Design review of the part built by this model. Coordinates are the model's own, in mm. Round coordinates to 2 decimals unless told otherwise and drop trailing zeros. Order: outer loops, then holes, each group sorted by start corner. A loop starts at its lowest first (then second) coordinate and runs counter-clockwise, first axis right, second up. Notation, with made-up numbers: M -16.75,36.5 L 16.25,36.5 A22 cw 16.25,74.5 Z; hole C -13,-10.5 d5. An arc over 180 degrees is marked long. Write item = value, one per line. Start each with the question number.
Autodesk Inventor part; units mm, degrees
ref_plane "YZ Plane" through (0, 0, 0) normal (1, 0, 0) x (0, 1, 0)
ref_plane "XZ Plane" through (0, 0, 0) normal (0, 1, 0) x (-1, 0, 0)
ref_plane "XY Plane" through (0, 0, 0) normal (0, 0, 1) x (1, 0, 0)
sketch "Sketch1" plane through (0, 0, 0) normal (0, 1, 0) x (-1, 0, 0)
  circle A0 centre (0, 0) radius 73.025
  line L0 (0, 0) -> (0, -73.025) construction
  line L1 (0, 0) -> (-12.6807, -71.9156)
  line L2 (0, 0) -> (12.6807, -71.9156)
  line L3 (0, 0) -> (72.3143, -10.1631)
  line L4 (0, 0) -> (64.4772, -34.2832)
  line L5 (0, 0) -> (32.0121, 65.6344)
  line L6 (0, 0) -> (52.5298, 50.7274)
  line L7 (0, 0) -> (-52.5298, 50.7274)
  line L8 (0, 0) -> (-32.0121, 65.6344)
  line L9 (0, 0) -> (-64.4772, -34.2832)
  line L10 (0, 0) -> (-72.3143, -10.1631)
  circle A1 centre (0, 0) radius 69.85
  arc A2 (4.7597, -69.6876) -> (-4.7597, -69.6876) centre (0, -69.85) ccw
  arc A3 (67.7477, -17.0079) -> (64.806, -26.0614) centre (66.4313, -21.5848) ccw
  arc A4 (37.1107, 59.1762) -> (44.8121, 53.5808) centre (41.0568, 56.5098) ccw
  arc A5 (-44.8121, 53.5808) -> (-37.1107, 59.1762) centre (-41.0568, 56.5098) ccw
  arc A6 (-64.806, -26.0614) -> (-67.7477, -17.0079) centre (-66.4313, -21.5848) ccw
  point P0 (61.6739, -32.7926)
  point P1 (69.1702, -9.7212)
  point P2 (50.2459, 48.5219)
  point P3 (30.6202, 62.7808)
  point P4 (-30.6202, 62.7808)
  point P5 (-50.2459, 48.5219)
  point P6 (-69.1702, -9.7212)
  point P7 (-61.6739, -32.7926)
  point P8 (-12.1293, -68.7888)
  point P9 (12.1293, -68.7888)
  point P10 (64.806, -26.0614)
  point P11 (67.7477, -17.0079)
  point P12 (44.8121, 53.5808)
  point P13 (37.1107, 59.1762)
  point P14 (-37.1107, 59.1762)
  point P15 (-67.7477, -17.0079)
  dimension "d0" = 146.05
  dimension "d1" = 10
  dimension "d4" = 360
  dimension "d6" = 3.175
  dimension "d10" = 9.525
  dimension "d13" = 360
extrude "Extrusion1" add sketch "Sketch1" along normal blind 1.5875 contours A0 L3 A1 L6 | L5 A1 L8 A0 | A1 L3 L6 | L6 L5 A1 A4 | A0 L2 A1 L4 | A1 A3 L4 L3 | L5 L8 A1 | L2 A1 A2 L1 | L4 A1 L2 | L10 A1 L7 | L7 A1 A5 L8 | L1 A1 L9 | L9 A1 A6 L10 | A0 L1 A1 L2 | L7 A1 L10 A0 | L1 A0 L9 A1 | A2 A1
fillet "Fillet1" radius 1.5875 24 edges at (30.6202, 0.7937, 62.7808) (32.0121, 0.7937, 65.6344) (-30.6202, 0.7937, 62.7808) (-32.0121, 0.7937, 65.6344) (-52.5298, 0.7937, 50.7274) (-50.2459, 0.7937, 48.5219) (52.5298, 0.7937, 50.7274) (50.2459, 0.7937, 48.5219) (64.4772, 0.7937, -34.2832) (61.6739, 0.7937, -32.7926) (72.3143, 0.7937, -10.1631) (69.1702, 0.7937, -9.7212) (-72.3143, 0.7937, -10.1631) (-69.1702, 0.7937, -9.7212) (-64.4772, 0.7937, -34.2832) (-61.6739, 0.7937, -32.7926) (37.1107, 0.7937, 59.1762) (44.8121, 0.7937, 53.5808) (-44.8121, 0.7937, 53.5808) (-37.1107, 0.7937, 59.1762) (-64.806, 0.7937, -26.0614) (-67.7477, 0.7937, -17.0079) (67.7477, 0.7937, -17.0079) (64.806, 0.7937, -26.0614)
sketch "Sketch5" plane through (0, 1.5875, 0) normal (0, 1, 0) x (1, 0, 0)
  line L0 (0, 0) -> (0, 65.0875) construction
  circle A0 centre (0, 50.8) radius 22.225
  arc A1 (63.6995, 35.7075) -> (-63.6995, 35.7075) centre (0, 0) ccw
  circle A2 centre (0, 50.8) radius 12.5 construction
  circle A3 centre (-24.6062, 60.325) radius 1.7526
  circle A4 centre (-24.6062, 60.325) radius 3.175 construction
  circle A5 centre (-22.225, 34.925) radius 3.175
  circle A6 centre (-22.225, 34.925) radius 1.7526
  circle A7 centre (24.6062, 60.325) radius 1.7526
  circle A8 centre (24.6062, 60.325) radius 3.175
  circle A9 centre (22.225, 34.925) radius 3.175
  circle A10 centre (22.225, 34.925) radius 1.7526
  arc A11 (-62.3874, 31.414) -> (-64.248, 27.4085) centre (0, 0) ccw
  arc A12 (63.6995, 35.7075) -> (-63.6995, 35.7075) centre (0, 0) ccw
  line L1 (-28.4451, 67.2572) -> (-25.3861, 34.6286)
  line L2 (-22.7046, 31.7864) -> (-3.3572, 28.83)
  line L3 (28.4451, 67.2572) -> (25.3861, 34.6286)
  line L4 (22.7046, 31.7864) -> (3.3572, 28.83)
  circle A13 centre (0, 63.3) radius 1.5
  circle A14 centre (-8.8388, 59.6388) radius 1.5
  circle A15 centre (-12.5, 50.8) radius 1.5
  circle A16 centre (-8.8388, 41.9612) radius 1.5
  circle A17 centre (0, 50.8) radius 6.35
  circle A18 centre (0, 0) radius 73.025
  circle A19 centre (0, 38.3) radius 1.5
  circle A20 centre (8.8388, 41.9612) radius 1.5
  circle A21 centre (12.5, 50.8) radius 1.5
  circle A22 centre (8.8388, 59.6388) radius 1.5
  point P0 (-63.6995, 35.7075)
  dimension "d39" = 25
  dimension "d40" = 44.45
  dimension "d41" = 3.5052
  dimension "d42" = 6.35
  dimension "d43" = 9.525
  dimension "d44" = 24.6062
  dimension "d45" = 6.35
  dimension "d46" = 3.5052
  dimension "d47" = 15.875
  dimension "d48" = 22.225
  dimension "d63" = 3
  dimension "d66" = 360
  dimension "d68" = 12.7
extrude "Extrusion3" cut sketch "Sketch5" against normal blind 25.4 contours A0 L4 A9 L3 A1 A18 L1 A5 L2 | A3 | A6 | A7 | A10 | A13 | A14 | A15 | A16 | A17 | A19 | A20 | A21 | A22
fillet "Fillet4" radius 6.35 2 edges at (-28.4451, 0.7937, -67.2572) (28.4451, 0.7937, -67.2572)
sketch "Sketch7" plane through (0, 1.5875, 0) normal (0, 1, 0) x (1, 0, 0)
  arc A0 (27.9955, 62.4615) -> (23.7373, 69.0593) centre (21.6732, 63.0542) ccw
  arc A1 (23.7373, 69.0593) -> (-23.7373, 69.0593) centre (0, 0) ccw
  arc A2 (-23.7373, 69.0593) -> (-27.9955, 62.4615) centre (-21.6732, 63.0542) ccw
  line L0 (-27.9955, 62.4615) -> (-25.3861, 34.6286)
  arc A3 (-25.3861, 34.6286) -> (-22.7046, 31.7864) centre (-22.225, 34.925) ccw
  line L1 (-22.7046, 31.7864) -> (-3.3572, 28.83)
  arc A4 (-3.3572, 28.83) -> (3.3572, 28.83) centre (0, 50.8) ccw
  line L2 (3.3572, 28.83) -> (22.7046, 31.7864)
  arc A5 (22.7046, 31.7864) -> (25.3861, 34.6286) centre (22.225, 34.925) ccw
  line L3 (25.3861, 34.6286) -> (27.9955, 62.4615)
  circle A6 centre (8.8388, 41.9612) radius 1.5
  circle A7 centre (-8.8388, 59.6388) radius 1.5
  circle A8 centre (22.225, 34.925) radius 1.7526
  circle A9 centre (-22.225, 34.925) radius 1.7526
  circle A10 centre (0, 63.3) radius 1.5
  circle A11 centre (12.5, 50.8) radius 1.5
  circle A12 centre (0, 38.3) radius 1.5
  circle A13 centre (0, 50.8) radius 6.35
  circle A14 centre (24.6062, 60.325) radius 1.7526
  circle A15 centre (-24.6062, 60.325) radius 1.7526
  circle A16 centre (-12.5, 50.8) radius 1.5
  circle A17 centre (-8.8388, 41.9612) radius 1.5
  circle A18 centre (8.8388, 59.6388) radius 1.5
  circle A19 centre (0, 50.8) radius 19.05
  line L4 (-18.9668, 49.0219) -> (-17.2732, 30.9565)
  line L5 (-3.3572, 28.83) -> (-22.7046, 31.7864)
  line L6 (-27.9955, 62.4615) -> (-25.3861, 34.6286)
  arc A20 (23.7373, 69.0593) -> (-23.7373, 69.0593) centre (0, 0) ccw
  line L7 (0, 73.025) -> (0, 28.575) construction
  line L8 (18.9668, 49.0219) -> (17.2732, 30.9565)
  dimension "d70" = 38.1
equation "\"d45\" = d42"
equation "\"d46\" = d41"
properties part number "Top Plate" material "Aluminum 6061"
(1) Consider section C-C, the plane x = -12.5. Write out the cut boundary in (y, z).
(2) Draft analysis for pull direction X (two halves, no side actions). For faces 1 (the face through (26.976, 0.783, -66.547)), 2 (the face through (-23.8, 0.8, -58.77)), 3 (the face through (-0.338, 0.783, -73.024)), state which applies: pulls with the +X half, pulls with the -X half, needs draft (parallel to the pull), parting line crosses it, or undercut.
(3) Consider section B-B, the plane z = -50.8. Write out the cut boundary in (x, y).
(4) Consider section D-D, the plane z = -63.3. Write out the cut boundary in (x, y), then the cut area to 3 significant figures.
(5) For line 1 along Z through (x, y) = (0, 0.4) (3 decimals); line 2 along Z through (x, y) = (8.5, 0.15); line 3 along X through (y, z) = (0.45, -61.5), list the stretches that pass through material, from the lowest coordinate up. Write a range as [from, to].
(6) Consider section A-A, the plane x = 0. State how many separate pieces and enclosed holes the cut face has, then the cut area to 3 significant figures.
(7) Insertion check: pin 1 (3 mm diameter, centred on x = -22.225, z = -34.925, fed in from +Y). The pin has a flat end and moves straight along its axis. Give the tip position at first contact, or say it passes through.
Completed:
q1.outline = M 0,-71.95 L 1.59,-71.95 L 1.59,-52.3 L 0,-52.3 Z; M 0,-49.3 L 1.59,-49.3 L 1.59,-30.23 L 0,-30.23 Z
q2.face_1 = pulls with the +X half
q2.face_2 = undercut
q2.face_3 = parting line crosses it
q3.outline = M -26.9,0 L -14,0 L -14,1.59 L -26.9,1.59 Z; M -11,0 L -6.35,0 L -6.35,1.59 L -11,1.59 Z; M 6.35,0 L 11,0 L 11,1.59 L 6.35,1.59 Z; M 14,0 L 26.9,0 L 26.9,1.59 L 14,1.59 Z
q4.outline = M -28.02,0 L -1.5,0 L -1.5,1.59 L -28.02,1.59 Z; M 1.5,0 L 28.02,0 L 28.02,1.59 L 1.5,1.59 Z
q4.area = 84.2 mm2
q5.line_1 = [-73.025, -64.8], [-61.8, -57.15], [-44.45, -39.8], [-36.8, -28.575]
q5.line_2 = [-72.53, -61.1], [-58.18, -43.42], [-40.5, -29.62]
q5.line_3 = [-27.91, -25.91], [-23.31, 23.31], [25.91, 27.91]
q6.separate_pieces = 4
q6.enclosed_holes = 0
q6.area = 40.9 mm2
q7.pin_1 = through
